Answer from the drawing. Dimensions are ordinates in mm from the lowest x, y and z of the part. Coordinates: 2 decimals unless noted, no trailing zeros. Loops run counter-clockwise (first coordinate to the right, second up) from the corner with the lowest first, then second, coordinate; pieces in that order, holes last. Notation, with made-up numbers: (-27, -13) - (-14, -13) arc R14 ccw to (-14, 3) - close; hole circle Ø4 at (76, 34). An arc over 180 degrees is marked (long way). Write each question's results on one line, items separated by ' | '. Start each with the question number.
1. A cutting plane is placed at C-C on x = 5. State how many separate pieces and enclosed holes the cut face has, then the cut area to 3 significant figures.
2. This flat-tipped pin is pushed along its axis until it touches: P1, Ø2.5, axis at y = 105, z = 5, coming from the -X side. Where does it stop, or does it pass through?
3. A cutting plane is placed at B-B on y = 80. Determine the outline of the cut face in (x, z) (3 decimals), then the cut area to 3 significant figures.
4. Find the intervals of material crossed by line 1 along Y through (x, z) = (5, 0.4) (3 decimals); line 2 along Y through (x, z) = (9.5, 5) (3 decimals); line 3 along Z through (x, y) = (2, 118), in increasing order. Write a range as [from, to].
5. A cutting plane is placed at A-A on z = 5. Determine the outline of the cut face in (x, y) (3 decimals).
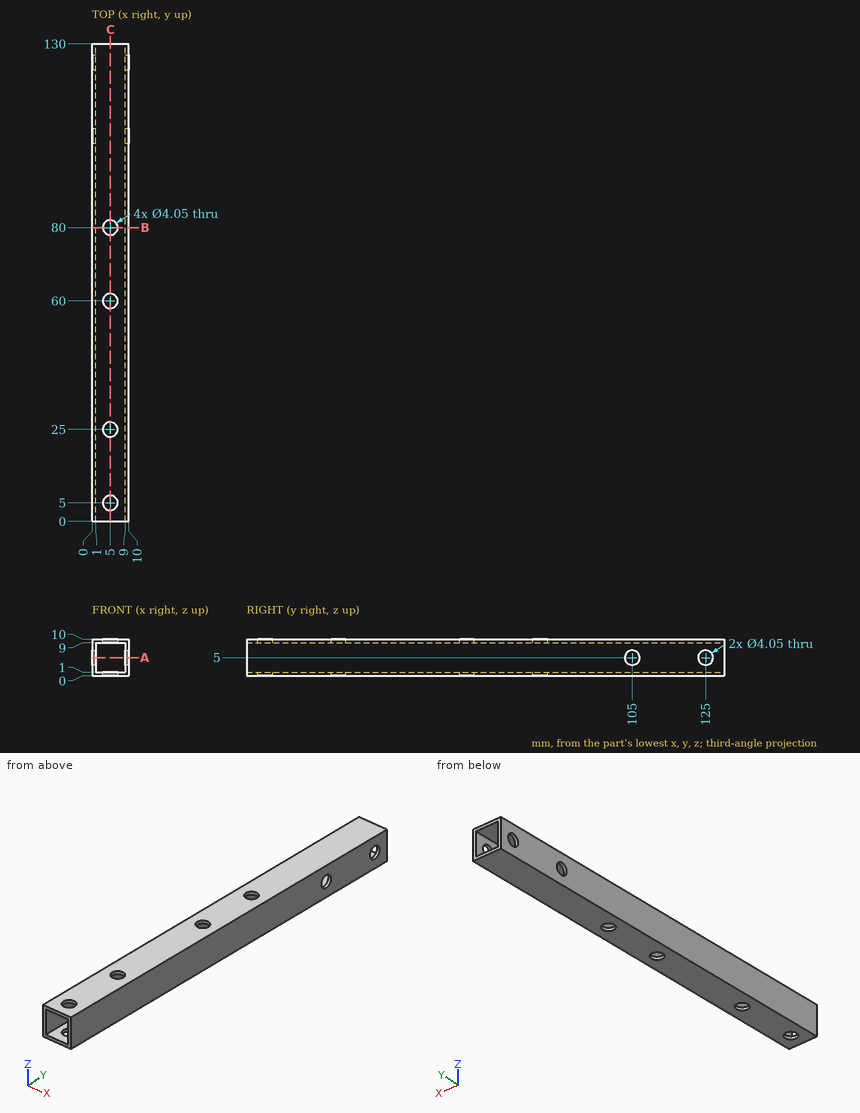
Values:
1) separate pieces: 10 | enclosed holes: 0 | area: 228 mm^2
2) P1: through
3) outline: (0, 0) - (2.975, 0) - (2.975, 1) - (1, 1) - (1, 9) - (2.975, 9) - (2.975, 10) - (0, 10) - close; (7.025, 0) - (10, 0) - (10, 10) - (7.025, 10) - (7.025, 9) - (9, 9) - (9, 1) - (7.025, 1) - close | area: 27.9 mm^2
4) line 1: [0, 2.975], [7.025, 22.975], [27.025, 57.975], [62.025, 77.975], [82.025, 130] | line 2: [0, 102.975], [107.025, 122.975], [127.025, 130] | line 3: [0, 1], [9, 10]
5) outline: (0, 0) - (1, 0) - (1, 102.975) - (0, 102.975) - close; (0, 107.025) - (1, 107.025) - (1, 122.975) - (0, 122.975) - close; (0, 127.025) - (1, 127.025) - (1, 130) - (0, 130) - close; (9, 0) - (10, 0) - (10, 102.975) - (9, 102.975) - close; (9, 107.025) - (10, 107.025) - (10, 122.975) - (9, 122.975) - close; (9, 127.025) - (10, 127.025) - (10, 130) - (9, 130) - close
